from build123d import *

# Parameters (mm, degrees)
F1_DEPTH = 5
F2_R     = 1.1
F3_DEPTH = 5.001
F4_R     = 1.5
F5_DEPTH = 5.001
F7_DEPTH = 5.001


with BuildPart() as f1:
    # F0 (on Top) → F1 (new body)
    with BuildSketch(Plane.XY):
        with BuildLine():
            ThreePointArc((146, 48), (145.12132, 50.12132), (143, 51))
            Line((143, 51), (-143, 51))
            ThreePointArc((-143, 51), (-145.12132, 50.12132), (-146, 48))
            Line((-146, 48), (-146, -48))
            ThreePointArc((-146, -48), (-145.12132, -50.12132), (-143, -51))
            Line((-143, -51), (143, -51))
            ThreePointArc((143, -51), (145.12132, -50.12132), (146, -48))
            Line((146, -48), (146, 48))
        make_face()
    extrude(amount=F1_DEPTH)

    # F2 (on face) → F3 (cut, through all)
    with BuildSketch(Plane.XY.offset(5)):
        with Locations((-142, 47)):
            Circle(F2_R)
        with Locations((142, 47)):
            Circle(F2_R)
        with Locations((-66.825193, 47)):
            Circle(F2_R)
        with Locations((66.174807, 47)):
            Circle(F2_R)
        with Locations((-142, -47)):
            Circle(F2_R)
        with Locations((142, -47)):
            Circle(F2_R)
        with Locations((-71, -47)):
            Circle(F2_R)
        with Locations((46, -47)):
            Circle(F2_R)
        with Locations((142, 3)):
            Circle(F2_R)
        with Locations((-142, 3)):
            Circle(F2_R)
    extrude(amount=-F3_DEPTH, mode=Mode.SUBTRACT)

    # F4 (on face) → F5 (cut, through all)
    with BuildSketch(Plane.XY.offset(5)):
        with BuildLine():
            Line((-71.407769, 47), (-137.417424, 47))
            ThreePointArc((-137.417424, 47), (-138.512869, 46.67332), (-139.250455, 45.8))
            ThreePointArc((-139.250455, 45.8), (-139.87868, 44.87868), (-140.8, 44.250455))
            ThreePointArc((-140.8, 44.250455), (-141.67332, 43.512869), (-142, 42.417424))
            Line((-142, 42.417424), (-142, 7.582576))
            ThreePointArc((-142, 7.582576), (-141.67332, 6.487131), (-140.8, 5.749545))
            ThreePointArc((-140.8, 5.749545), (-139, 3), (-140.8, 0.250455))
            ThreePointArc((-140.8, 0.250455), (-141.67332, -0.487131), (-142, -1.582576))
            Line((-142, -1.582576), (-142, -42.417424))
            ThreePointArc((-142, -42.417424), (-141.67332, -43.512869), (-140.8, -44.250455))
            ThreePointArc((-140.8, -44.250455), (-139.87868, -44.87868), (-139.250455, -45.8))
            ThreePointArc((-139.250455, -45.8), (-138.512869, -46.67332), (-137.417424, -47))
            Line((-137.417424, -47), (-75.582576, -47))
            ThreePointArc((-75.582576, -47), (-74.487131, -46.67332), (-73.749545, -45.8))
            ThreePointArc((-73.749545, -45.8), (-71, -44), (-68.250455, -45.8))
            ThreePointArc((-68.250455, -45.8), (-67.512869, -46.67332), (-66.417424, -47))
            Line((-66.417424, -47), (41.417424, -47))
            ThreePointArc((41.417424, -47), (42.512869, -46.67332), (43.250455, -45.8))
            ThreePointArc((43.250455, -45.8), (46, -44), (48.749545, -45.8))
            ThreePointArc((48.749545, -45.8), (49.487131, -46.67332), (50.582576, -47))
            Line((50.582576, -47), (137.417424, -47))
            ThreePointArc((137.417424, -47), (138.512869, -46.67332), (139.250455, -45.8))
            ThreePointArc((139.250455, -45.8), (139.87868, -44.87868), (140.8, -44.250455))
            ThreePointArc((140.8, -44.250455), (141.67332, -43.512869), (142, -42.417424))
            Line((142, -42.417424), (142, -1.582576))
            ThreePointArc((142, -1.582576), (141.67332, -0.487131), (140.8, 0.250455))
            ThreePointArc((140.8, 0.250455), (139, 3), (140.8, 5.749545))
            ThreePointArc((140.8, 5.749545), (141.67332, 6.487131), (142, 7.582576))
            Line((142, 7.582576), (142, 42.417424))
            ThreePointArc((142, 42.417424), (141.67332, 43.512869), (140.8, 44.250455))
            ThreePointArc((140.8, 44.250455), (139.87868, 44.87868), (139.250455, 45.8))
            ThreePointArc((139.250455, 45.8), (138.512869, 46.67332), (137.417424, 47))
            Line((137.417424, 47), (109.757383, 47))
            ThreePointArc((109.757383, 47), (108.661938, 46.67332), (107.924352, 45.8))
            ThreePointArc((107.924352, 45.8), (105.174807, 44), (102.425262, 45.8))
            ThreePointArc((102.425262, 45.8), (101.687676, 46.67332), (100.592231, 47))
            Line((100.592231, 47), (70.757383, 47))
            ThreePointArc((70.757383, 47), (69.661938, 46.67332), (68.924352, 45.8))
            ThreePointArc((68.924352, 45.8), (66.174807, 44), (63.425262, 45.8))
            ThreePointArc((63.425262, 45.8), (62.687676, 46.67332), (61.592231, 47))
            Line((61.592231, 47), (-62.242617, 47))
            ThreePointArc((-62.242617, 47), (-63.338062, 46.67332), (-64.075648, 45.8))
            ThreePointArc((-64.075648, 45.8), (-66.825193, 44), (-69.574738, 45.8))
            ThreePointArc((-69.574738, 45.8), (-70.312324, 46.67332), (-71.407769, 47))
        make_face()
        with Locations((-142, 47)):
            Circle(F4_R)
        with Locations((-66.825193, 47)):
            Circle(F4_R)
        with Locations((-142, 3)):
            Circle(F4_R)
        with Locations((-142, -47)):
            Circle(F4_R)
        with Locations((66.174807, 47)):
            Circle(F4_R)
        with Locations((142, 3)):
            Circle(F4_R)
        with Locations((142, -47)):
            Circle(F4_R)
        with Locations((46, -47)):
            Circle(F4_R)
        with Locations((-71, -47)):
            Circle(F4_R)
        with Locations((142, 47)):
            Circle(F4_R)
        with Locations((105.174807, 47)):
            Circle(F4_R)
    extrude(amount=-F5_DEPTH, mode=Mode.SUBTRACT)

    # F6 (on face) → F7 (cut, through all)
    with BuildSketch(Plane.XY.offset(5)):
        Polygon((89.5, 51), (82.5, 51), (82.5, 49), (77, 49), (77, 47), (95, 47), (95, 49), (89.5, 49), align=None)
    extrude(amount=-F7_DEPTH, mode=Mode.SUBTRACT)


solid = f1.part
CAD build for the part. Positions are in the model's coordinates, mm. A direction names the side the tool comes from. Round coordinates to 2 decimals unless told otherwise and drop trailing zeros. Write each loop counter-clockwise with the first axis right and the second up, starting at its lowest first coordinate (ties: lowest second). Pieces come first, ordered by that corner, then holes.
(1) Slice it at C-C, the plane z = 3.6. Count the separate pieces of the cut face and the enclosed holes in it, and give its area (3 significant figures).
(2) 3-axis set-ups, long thin cutter, end or side, ignore diameter. For faces 1 (the face through (74, 47, 3)), 2 (the face through (-1, 49, 5)): which of +Z, -Z, +X, -X, +Y, -Y reach the whole face in a straight line?
(3) Probe line 1 along Y through (x, z) = (-43.5, 4.2); line 2 along Y through (x, z) = (90.5, 3.8); line 3 along X through (y, z) = (-15.5, 2.05). List the from-to ranges inside material, lowest first.
(4) Slice it at A-A, the plane x = -107. Write the cut outline in (y, z).
(5) Slice it at B-B, the plane y = -8. Write the cut outline in (x, z), and give its area (3 significant figures).
(6) Drop flat-ended pins along their axis: P1, Ø2.5, axis at x = 46, y = -47, coming from the -Z side; P2, Ø5, axis at x = -71, y = -47, coming from the -Z side; P3, Ø1.6, axis at y = 49.5, z = 2, coming from the -X side; P4, Ø1.6, axis at y = 49.5, z = 2.5, coming from the +X side. Give the stop position or say it passes through.
(7) Mould opens along X. For faces 3 (the face through (-66.8, 44, 2.5)), 4 (the face through (117, 51, 2)), 5 (the face through (146, -1, 2)) say: pulls with the +X half, pulls with the -X half, needs draft (parallel to the pull), parting line crosses it, or undercut.
From the geometry:
1. separate pieces: 1
1. enclosed holes: 11
1. area: 3,090 mm2
2. face 1: +Z, -Z
2. face 2: +Z, +X, -X, +Y, -Y
3. line 1: y = -51 to -47, 47 to 51
3. line 2: y = -51 to -47, 49 to 51
3. line 3: x = -146 to -142, 142 to 146
4. outline: (-51, 0) - (-47, 0) - (-47, 5) - (-51, 5) - close; (47, 0) - (51, 0) - (51, 5) - (47, 5) - close
5. outline: (-146, 0) - (-142, 0) - (-142, 5) - (-146, 5) - close; (142, 0) - (146, 0) - (146, 5) - (142, 5) - close
5. area: 40.0 mm2
6. P1: passes through
6. P2: stops at z = 0
6. P3: stops at x = -145.92
6. P4: stops at x = 145.92
7. face 3: undercut
7. face 4: needs draft
7. face 5: pulls with the +X half
